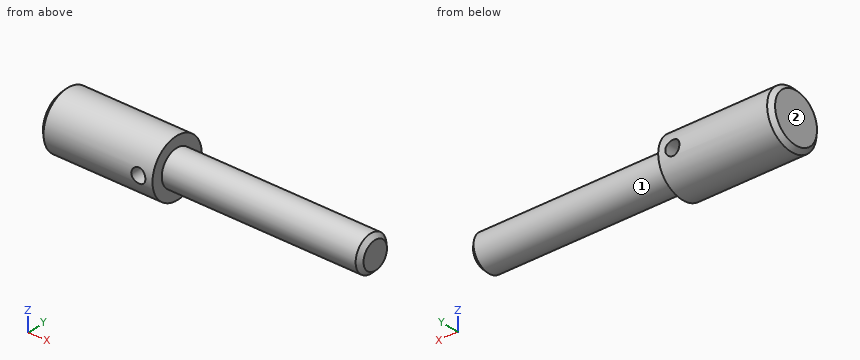
from build123d import *

# Parameters (mm, degrees)
CHAMFER_1_SIZE           = 0.6
CUT_EXTRUDE_1_REACH      = 46.9
CUT_EXTRUDE_1_END_RADIUS = 4
SKETCH_2_R               = 1


with BuildPart() as part:
    # Эскиз1 → Повернуть1 (revolve)
    with BuildSketch(Plane.XY):
        Polygon((0, 0), (16, 0), (16, -1.5), (44, -1.5), (44, -4), (0, -4), align=None)
    revolve(axis=Axis((44, -4, 0), (-1, 0, 0)))

    # Фаска1
    chamfer_1_edges = [part.edges().sort_by_distance(p)[0] for p in [
        (44, -6.5, 0),
        (0, -8, 0),
    ]]
    chamfer(chamfer_1_edges, length=CHAMFER_1_SIZE)

    # Вырез-Вытянуть1: up to this cylinder (the profile starts inside it)
    cut_extrude_1_end = Plane(origin=(14, -4, 0), z_dir=(1, 0, 0)) * Cylinder(CUT_EXTRUDE_1_END_RADIUS, 102.8, mode=Mode.PRIVATE)
    # Эскиз2 → Вырез-Вытянуть1 (cut, up to the surface)
    with BuildSketch(Plane(origin=(0, 0, 0), x_dir=(1, 0, 0), z_dir=(0, 1, 0)), mode=Mode.PRIVATE) as cut_extrude_1_sk1:
        with Locations(Location((14, 0, 0), (0, 0, 270))):
            Circle(SKETCH_2_R)
    cut_extrude_1_tool1 = extrude(cut_extrude_1_sk1.sketch, amount=-CUT_EXTRUDE_1_REACH, mode=Mode.PRIVATE) & cut_extrude_1_end
    add(cut_extrude_1_tool1.solids().sort_by_distance((14, 0, 0))[0], mode=Mode.SUBTRACT)


solid = part.part
CAD build for the part. Positions are in the model's coordinates, mm. Face numbers are marked on the shaded views. A direction names the side the tool comes from. Coordinates: 2 decimals unless noted, no trailing zeros. Loops run counter-clockwise (first coordinate to the right, second up) from the corner with the lowest first, then second, coordinate; pieces in that order, holes last. Notation, with made-up numbers: (76.25, -26) -> (108.25, -26) arc R20 ccw to (108.25, 4) -> close; hole circle Ø2 at (-35, 16.25). An arc over 180 degrees is marked (long way). One line per item, written item: value.
1. Slice it at B-B on y = -4. Write the cut outline in (x, z), and give its area (3 significant figures).
Answers:
outline: (0, -3.4) -> (0.6, -4) -> (16, -4) -> (16, -2.5) -> (43.4, -2.5) -> (44, -1.9) -> (44, 1.9) -> (43.4, 2.5) -> (16, 2.5) -> (16, 4) -> (0.6, 4) -> (0, 3.4) -> close; hole circle Ø2 at (14, 0)
area: 264 mm^2
2. Flat gauge pins, fed straight in: P1, Ø3, axis at x = 24.5, y = -5, coming from the -Z side; P2, Ø4, axis at y = -5.5, z = 2, coming from the +X side; P3, Ø1.5, axis at x = 27.5, z = 3, coming from the -Y side. Where does each tip first touch, or does it go through?
Answers:
P1: stops at z = -2.5
P2: stops at x = 44
P3: stops at y = -5.09
3. Slice it at C-C on x = 7. Write the cut outline in (y, z), and give its area (3 significant figures).
Answers:
outline: circle Ø8 at (-4, 0)
area: 50.3 mm^2
4. Slice it at A-A on z = 0. Write the cut outline in (x, y), and give its area (3 significant figures).
Answers:
outline: (0, -7.4) -> (0.6, -8) -> (13, -8) -> (13, 0) -> (0.6, 0) -> (0, -0.6) -> close; (15, -8) -> (16, -8) -> (16, -6.5) -> (43.4, -6.5) -> (44, -5.9) -> (44, -2.1) -> (43.4, -1.5) -> (16, -1.5) -> (16, 0) -> (15, 0) -> close
area: 251 mm^2
5. Drill centre lines: line 1 (X direction, y = -1.25, z = 0); line 2 (X direction, y = -2.5, z = 0); line 3 (Z direction, x = 4, y = -4.25). Where is each one in solid material? Low to high. Write a range as [from, to].
Answers:
line 1: x = [0, 13], [15, 16]
line 2: x = [0, 13], [15, 44]
line 3: z = [-3.99, 3.99]
6. Slice it at D-D on x = 13.5. Write the cut outline in (y, z), and give its area (3 significant figures).
Answers:
outline: (-7.91, -0.87) arc R4 ccw to (-0.09, -0.87) -> close; (-7.91, 0.87) -> (-0.09, 0.87) arc R4 ccw to start
area: 36.5 mm^2
7. Which spindle directions (+Z, -Z, +X, -X, +Y, -Y) get a long thin tool onto all of the face, cutting with end or side? Do the marked faces 1 and 2. Say none if no direction does.
Answers:
face 1: +X
face 2: +Z, -Z, -X, +Y, -Y
